Could you check a few things on this model? Use its own coordinates, in mm. Face numbers are marked on the shaded views. A direction names the side the tool comes from. Round coordinates to 2 decimals unless told otherwise and drop trailing zeros. Loops run counter-clockwise (first coordinate to the right, second up) from the corner with the lowest first, then second, coordinate; pieces in that order, holes last. Notation, with made-up numbers: (39.25, 67.25) -> (85.25, 67.25) arc R21 ccw to (85.25, 84.25) -> close; hole circle Ø5 at (43.25, 86). An arc over 180 degrees is marked (long way). One line per item, written item: value.
Autodesk Inventor part; units mm, degrees
ref_plane "YZ Plane" through (0, 0, 0) normal (1, 0, 0) x (0, 1, 0)
ref_plane "XZ Plane" through (0, 0, 0) normal (0, 1, 0) x (-1, 0, 0)
ref_plane "XY Plane" through (0, 0, 0) normal (0, 0, 1) x (1, 0, 0)
sketch "スケッチ1" plane through (0, 0, 0) normal (0, 1, 0) x (-1, 0, 0)
  line L0 (5.05, 2.05) -> (-5.05, 2.05)
  line L1 (-5.05, 2.05) -> (-5.05, -2.05)
  line L2 (-5.05, -2.05) -> (5.05, -2.05)
  line L3 (5.05, -2.05) -> (5.05, 2.05)
  line L4 (5.05, 2.05) -> (-5.05, -2.05) construction
  line L5 (-5.05, 2.05) -> (5.05, -2.05) construction
  line L6 (7.5, 4.6151) -> (-7.5, 4.6151)
  line L7 (-7.5, 4.6151) -> (-7.5, -4.6151)
  line L8 (-7.5, -4.6151) -> (7.5, -4.6151)
  line L9 (7.5, -4.6151) -> (7.5, 4.6151)
  line L10 (7.5, 4.6151) -> (-7.5, -4.6151) construction
  line L11 (-7.5, 4.6151) -> (7.5, -4.6151) construction
  point P0 (0, 0)
  dimension "d0" = 10.1
  dimension "d1" = 4.1
  dimension "d2" = 15
extrude "押し出し1" add sketch "スケッチ1" along normal blind 4
sketch "スケッチ2" plane through (0, 0, 0) normal (0, -1, 0) x (1, 0, 0)
  line L0 (7.5, 4.6151) -> (7.5, -4.6151)
  line L1 (-7.5, -4.6151) -> (7.5, -4.6151)
  line L2 (7.5, -4.6151) -> (7.5, -2.0651)
  line L3 (7.5, -2.0651) -> (-7.5, -2.0651)
  line L4 (-7.5, -2.0651) -> (-7.5, -4.6151)
  point P0 (0, 0)
  dimension "d5" = 2.55
extrude "押し出し2" add sketch "スケッチ2" along normal blind 6
sketch "スケッチ3" plane through (-7.5, 0, -2.0651) normal (0, 0, 1) x (1, 0, 0)
  line L0 (15, -6) -> (0, -6)
  line L1 (15, -6) -> (15, 4)
  line L2 (0, -6) -> (15, -6)
  line L3 (15, -6) -> (15, -3.5)
  line L4 (15, -3.5) -> (0, -3.5)
  line L5 (0, -3.5) -> (0, -6)
  point P0 (7.5, 0)
  dimension "d8" = 2.5
extrude "押し出し3" add sketch "スケッチ3" along normal blind 12.45
sketch "スケッチ4" plane through (-7.5, -3.5, -2.0651) normal (0, 1, 0) x (1, 0, 0)
  line L0 (1.5, 1.0597) -> (13.5, 1.0597)
  line L1 (13.5, 1.0597) -> (13.5, -5.1899)
  line L2 (13.5, -5.1899) -> (1.5, -5.1899)
  line L3 (1.5, -5.1899) -> (1.5, 1.0597)
  line L4 (1.5, 1.0597) -> (13.5, -5.1899) construction
  line L5 (13.5, 1.0597) -> (1.5, -5.1899) construction
  line L6 (1.5, -0.0039) -> (13.5, 0)
  line L7 (0, 0) -> (15, 0)
  point P0 (7.5, -2.0651)
  dimension "d11" = 12
extrude "押し出し4" cut sketch "スケッチ4" against normal blind 10 contours L1 L2 L3 L6
fillet "フィレット1" radius 2 4 edges at (7.5, -4.75, 10.3849) (-7.5, -4.75, 10.3849) (-7.5, -1, -4.6151) (7.5, -1, -4.6151)
properties part number "LRA_case2"
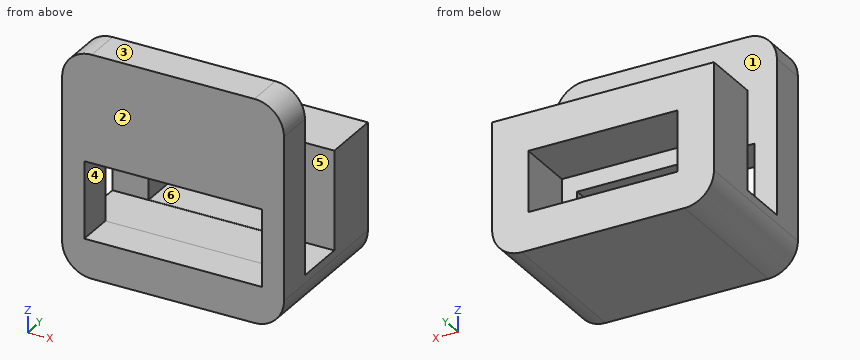
Item 1: If we mould it in two halves opening along Y, with no side actions, what happens to the marked faces 1, 2 and 3? For each: released by +Y, released by -Y, zero draft, split by the parting line, or undercut.
Output:
face 1: undercut
face 2: released by -Y
face 3: zero draft
Item 2: If we section it at D-D on x = 3.5: Count the separate pieces of the cut face and the enclosed holes in it, plus the area to 3 significant figures.
Output:
separate pieces: 3
enclosed holes: 0
area: 54.0 mm²
Item 3: I need wall thicknesses on line 1 (X direction, y = 2.75, z = 0); line 2 (Z direction, x = -4.5, y = -4.5); line 3 (Y direction, x = -3.25, z = 3.75). Which ranges of each line are inside material? Lowest first, please. Write a range as from..to.
Output:
line 1: x = -7.5..-5.05, 5.05..7.5
line 2: z = -4.62..-2.06, 3.12..10.38
line 3: y = -6..-3.5, 0..4
Item 4: If we section it at B-B on z = 0.75: List the corners of the cut face in (x, y) for me.
Output:
outline: (-7.5, -6) -> (-6, -6) -> (-6, -3.5) -> (-7.5, -3.5) -> close; (-7.5, 0) -> (-5.05, 0) -> (-5.05, 4) -> (-7.5, 4) -> close; (5.05, 0) -> (7.5, 0) -> (7.5, 4) -> (5.05, 4) -> close; (6, -6) -> (7.5, -6) -> (7.5, -3.5) -> (6, -3.5) -> close
Item 5: For the marked faces 4, 5 and 6, which set-ups out of +Z, -Z, +X, -X, +Y, -Y let a thin tool reach every point of the face, with its end or its side?
Output:
face 4: -Y
face 5: +Z, +X, -X
face 6: +Y, -Y
Item 6: If we section it at A-A on y = -5.25: List the corners of the cut face in (x, z) for me, plus the area to 3 significant figures.
Output:
outline: (-7.5, -2.62) arc R2 ccw to (-5.5, -4.62) -> (5.5, -4.62) arc R2 ccw to (7.5, -2.62) -> (7.5, 8.38) arc R2 ccw to (5.5, 10.38) -> (-5.5, 10.38) arc R2 ccw to (-7.5, 8.38) -> close; hole (-6, -2.06) -> (6, -2.07) -> (6, 3.12) -> (-6, 3.12) -> close
area: 159 mm²
Item 7: Will these pins go through, and if not, where does the flat tip stop? pin 1 Ø1 at (x, y) = (-3, -2) entering from +Z; pin 2 Ø1 at (x, z) = (-5.5, 7.5) entering from +Y; pin 3 Ø6 at (x, z) = (-3, 6.5) entering from +Y; pin 4 Ø5 at (x, y) = (-1.5, 1.5) entering from +Z.
Output:
pin 1: stops at z = -2.07
pin 2: stops at y = -3.5
pin 3: stops at y = 4
pin 4: stops at z = 4.62
